Geometry check sheet. Reference: the model listing, model coordinates, mm. A direction names the side the tool comes from. Coordinates: 2 decimals unless noted, no trailing zeros. Write each loop counter-clockwise with the first axis right and the second up, starting at its lowest first coordinate (ties: lowest second). Pieces come first, ordered by that corner, then holes. Notation, with made-up numbers: (-17.5, 82.5) -> (18.5, 82.5) arc R21 ccw to (18.5, 94.5) -> close; hole circle Ø5 at (-30, 34.25). An arc over 180 degrees is marked (long way). Answer as CSV lines item,"result".
```python
from build123d import *

# Parameters (mm, degrees)
BOSS_EXTRUDE1_DEPTH = 150
SKETCH3_R           = 4.25
SKETCH3_R_2         = 3.2
CUT_EXTRUDE1_DEPTH  = 170.558249578
SKETCH4_R           = 2
CUT_EXTRUDE2_DEPTH  = 166.858373319
SKETCH5_R           = 3.5
CUT_EXTRUDE3_DEPTH  = 5


with BuildPart() as part:
    # Sketch2 → Boss-Extrude1 (new body)
    with BuildSketch(Plane.XY):
        Polygon((0, 0), (0, 45), (65, 45), (65, 28), (20, 28), (20, 0), align=None)
    extrude(amount=BOSS_EXTRUDE1_DEPTH)

    # Sketch3 → Cut-Extrude1 (cut, through all)
    with BuildSketch(Plane.ZY):
        with Locations((17.5, 19)):
            Circle(SKETCH3_R)
        with Locations((132.5, 19)):
            Circle(SKETCH3_R)
        with Locations((75, 13)):
            Circle(SKETCH3_R)
        with Locations((37, 35)):
            Circle(SKETCH3_R_2)
        with Locations((113, 35)):
            Circle(SKETCH3_R_2)
    extrude(amount=-CUT_EXTRUDE1_DEPTH, mode=Mode.SUBTRACT)

    # Sketch4 → Cut-Extrude2 (cut, through all)
    with BuildSketch(Plane(origin=(0, 28, 0), x_dir=(1, 0, 0), z_dir=(0, 1, 0))):
        with Locations(Location((42.5, -29.5, 0), (0, 0, 180))):
            Circle(SKETCH4_R)
        with Locations(Location((42.5, -5.5, 0), (0, 0, 180))):
            Circle(SKETCH4_R)
        with Locations(Location((25.5, -5.5, 0), (0, 0, 180))):
            Circle(SKETCH4_R)
        with Locations(Location((25.5, -29.5, 0), (0, 0, 180))):
            Circle(SKETCH4_R)
        with Locations((42.5, -144.5)):
            Circle(SKETCH4_R)
        with Locations((42.5, -120.5)):
            Circle(SKETCH4_R)
        with Locations((25.5, -120.5)):
            Circle(SKETCH4_R)
        with Locations((25.5, -144.5)):
            Circle(SKETCH4_R)
        with Locations(Location((42.5, -87, 0), (0, 0, 180))):
            Circle(SKETCH4_R)
        with Locations(Location((42.5, -63, 0), (0, 0, 180))):
            Circle(SKETCH4_R)
        with Locations(Location((25.5, -63, 0), (0, 0, 180))):
            Circle(SKETCH4_R)
        with Locations(Location((25.5, -87, 0), (0, 0, 180))):
            Circle(SKETCH4_R)
    extrude(amount=CUT_EXTRUDE2_DEPTH, mode=Mode.SUBTRACT)

    # Sketch5 → Cut-Extrude3 (cut)
    with BuildSketch(Plane(origin=(0, 45, 0), x_dir=(1, 0, 0), z_dir=(0, 1, 0))):
        with Locations(Location((25.5, -5.5, 0), (0, 0, 270))):
            Circle(SKETCH5_R)
        with Locations(Location((42.5, -5.5, 0), (0, 0, 270))):
            Circle(SKETCH5_R)
        with Locations(Location((25.5, -29.5, 0), (0, 0, 270))):
            Circle(SKETCH5_R)
        with Locations(Location((42.5, -29.5, 0), (0, 0, 270))):
            Circle(SKETCH5_R)
        with Locations(Location((25.5, -63, 0), (0, 0, 270))):
            Circle(SKETCH5_R)
        with Locations(Location((42.5, -63, 0), (0, 0, 270))):
            Circle(SKETCH5_R)
        with Locations(Location((25.5, -87, 0), (0, 0, 270))):
            Circle(SKETCH5_R)
        with Locations(Location((42.5, -87, 0), (0, 0, 270))):
            Circle(SKETCH5_R)
        with Locations(Location((25.5, -120.5, 0), (0, 0, 270))):
            Circle(SKETCH5_R)
        with Locations(Location((42.5, -120.5, 0), (0, 0, 270))):
            Circle(SKETCH5_R)
        with Locations(Location((42.5, -144.5, 0), (0, 0, 270))):
            Circle(SKETCH5_R)
        with Locations(Location((25.5, -144.5, 0), (0, 0, 270))):
            Circle(SKETCH5_R)
    extrude(amount=-CUT_EXTRUDE3_DEPTH, mode=Mode.SUBTRACT)


solid = part.part
```
Item 1: Release check for a two-part mould opening along X. For faces 1 (the cylindrical face through (43.575, 33.916, 118.814)), 2 (the cylindrical face through (32.045, 35.961, 116.052)), 3 (the flat face through (65, 37, 74)) record: +X half, -X half, draft (parallel to the pull), parting line (faces both ways), or undercut.
Responses:
face 1,"undercut"
face 2,"draft"
face 3,"+X half"
Item 2: Cross-section at B-B, the plane x = 5. Record the cut outline in (y, z).
Responses:
outline,"(0, 0) -> (45, 0) -> (45, 150) -> (0, 150) -> close; hole circle Ø8.5 at (13, 75); hole circle Ø8.5 at (19, 17.5); hole circle Ø8.5 at (19, 132.5); hole circle Ø6.4 at (35, 37); hole circle Ø6.4 at (35, 113)"
Item 3: Depth check by flat-ended pin: pin 1 Ø6.5 at (x, z) = (25.5, 87) entering from -Y; pin 2 Ø8 at (x, y) = (19.5, 26.5) entering from -Z; pin 3 Ø3.5 at (x, z) = (43, 85.5) entering from +Y; pin 4 Ø1 at (y, z) = (14, 57.5) entering from +X. Enter the tip coordinate at first touch or a pass-through.
Responses:
pin 1,"stops at y = 28"
pin 2,"stops at z = 0"
pin 3,"stops at y = 40"
pin 4,"stops at x = 20"
Item 4: Cross-section at A-A, the plane z = 120.5. Record the cut outline in (x, y), plus the area to 3 significant figures.
Responses:
outline,"(0, 0) -> (20, 0) -> (20, 28) -> (23.5, 28) -> (23.5, 40) -> (22, 40) -> (22, 45) -> (0, 45) -> close; (27.5, 28) -> (40.5, 28) -> (40.5, 40) -> (39, 40) -> (39, 45) -> (29, 45) -> (29, 40) -> (27.5, 40) -> close; (44.5, 28) -> (65, 28) -> (65, 45) -> (46, 45) -> (46, 40) -> (44.5, 40) -> close"
area,"1,500 mm2"
Item 5: Set-up check for faces 4 (the cylindrical face through (42.76, 33.916, 88.983)), 5 (the cylindrical face through (28.45, 42.54, 7.38)), 6 (the flat face through (43, 28, 74)): record each of +Z, -Z, +X, -X, +Y, -Y from which the full face is reachable in a straight line by a thin tool's end or side.
Responses:
face 4,"+Y, -Y"
face 5,"+Y"
face 6,"+Z, -Z, +X, -Y"
Item 6: Cross-section at C-C, the plane y = 19. Record the cut outline in (x, z).
Responses:
outline,"(0, 0) -> (20, 0) -> (20, 13.25) -> (0, 13.25) -> close; (0, 21.75) -> (20, 21.75) -> (20, 128.25) -> (0, 128.25) -> close; (0, 136.75) -> (20, 136.75) -> (20, 150) -> (0, 150) -> close"
Item 7: Thickness scan on probe 1 along X at (y, z) = (35.25, 29.5); probe 2 along X at (y, z) = (42.6, 29.5); probe 3 along Z at (x, y) = (59, 34). Record the ranges inside material, lowest first.
Responses:
probe 1,"x = 0 to 23.5, 27.5 to 40.5, 44.5 to 65"
probe 2,"x = 0 to 22, 29 to 39, 46 to 65"
probe 3,"z = 0 to 33.96, 40.04 to 109.96, 116.04 to 150"
Item 8: Cross-section at D-D, the plane x = 42.5. Count the separate pieces of the cut face and the enclosed holes in it, plus the area to 3 significant figures.
Responses:
separate pieces,"7"
enclosed holes,"2"
area,"1,990 mm2"
